Source: CAD feature listing. Evaluate the final solid. Frame: model axes, mm. Coordinates: 2 decimals unless noted, no trailing zeros. Order: outer loops, then holes, each group sorted by start corner. A loop starts at its lowest first (then second) coordinate and runs counter-clockwise, first axis right, second up.
```python
from build123d import *

# Parameters (mm, degrees)
CROQUIS2_R              = 2.6
SALIENTE_EXTRUIR2_DEPTH = 20


with BuildPart() as part:
    # Croquis2 → Saliente-Extruir2 (new body)
    with BuildSketch(Plane.XY):
        with BuildLine():
            Line((5, 0), (5, 25))
            Line((5, 25), (0, 25))
            Line((0, 25), (-10, 25))
            Line((-10, 25), (-10, -5))
            Line((-10, -5), (0, -5))
            ThreePointArc((0, -5), (3.535533906, -3.535533906), (5, 0))
        make_face()
        Circle(CROQUIS2_R, mode=Mode.SUBTRACT)
    extrude(amount=SALIENTE_EXTRUIR2_DEPTH)


solid = part.part
```
1. Section query B-B, the plane y = -0.5. Output: boundary loops of the cut face in (x, z), plus the area to 3 significant figures.
2. Draft query along X for faces 1 (the flat face through (-10, 10, 10)), 2 (the flat face through (-3, 10, 0)), 3 (the cylindrical face through (-0.338, 2.578, 9.86)), 4 (the cylindrical face through (3, -4, 10)). Return one class per face: +X half, -X half, draft (parallel to the pull), parting line (faces both ways), or undercut.
3. Material intervals for line 1 along Y through (x, z) = (0, 8.75); line 2 along X through (y, z) = (-1, 7.75); line 3 along Y through (x, z) = (4, 7.75), sorted ascending.
4. Section query C-C, the plane x = 4. Output: boundary loops of the cut face in (y, z), plus the area to 3 significant figures.
5. Contact query for a flat-ended pin moving along its axis: P1, Ø3, axis at x = 0, y = 0, coming from the +Z side. Output: stop coordinate, or through.
6. Section query A-A, the plane z = 2.5. Output: boundary loops of the cut face in (x, y), plus the area to 3 significant figures.
Answer key:
1. outline: (-10, 0) - (-2.55, 0) - (-2.55, 20) - (-10, 20) - close; (2.55, 0) - (4.97, 0) - (4.97, 20) - (2.55, 20) - close
1. area: 197 mm2
2. face 1: -X half
2. face 2: draft
2. face 3: undercut
2. face 4: +X half
3. line 1: y = -5 to -2.6, 2.6 to 25
3. line 2: x = -10 to -2.4, 2.4 to 4.9
3. line 3: y = -3 to 25
4. outline: (-3, 0) - (25, 0) - (25, 20) - (-3, 20) - close
4. area: 560 mm2
5. P1: passes through
6. outline: (-10, -5) - (0, -5) arc R5 ccw to (5, 0) - (5, 25) - (-10, 25) - close; hole circle Ø5.2 at (0, 0)
6. area: 423 mm2
